Print and shaded views of the part. All mm, measured from the part's lowest x, y and z. A direction names the side the tool comes from. Coordinates: 2 decimals unless noted, no trailing zeros. Loops run counter-clockwise (first coordinate to the right, second up) from the corner with the lowest first, then second, coordinate; pieces in that order, holes last. Notation, with made-up numbers: (-16, -31) -> (1, -31) arc R17 cw to (1, -13) -> close; hole circle Ø4 at (-35, 44.5). An arc over 180 degrees is marked (long way). One line per question, with ' | ' between items. Start each with the question number.
1) Two-plate mould, pull along Z, no slides. Class the marked faces 1, 2 and 3: released by +Z, released by -Z, zero draft, split by the parting line, or undercut.
2) Probe L1, parallel to Y at x = 2.5, z = 6.25; L2, parallel to Z at x = 2.75, y = 3.4; L3, parallel to Z at x = 4.5, y = 2.85. List the from-to ranges inside material, lowest first. Write a range as from..to.
3) Cut at A-A (x = 3.5). List the corners of the cut face in (y, z), plus the area to 3 significant figures.
4) 3-axis set-ups, long thin cutter, end or side, ignore diameter. For the marked faces 4 and 5: which of +Z, -Z, +X, -X, +Y, -Y reach the whole face in a straight line?
5) Cut at B-B (y = 2.35). List the corners of the cut face in (x, z).
6) Cut at D-D (x = 1). List the corners of the cut face in (y, z).
7) Cut at C-C (z = 3.25). List the corners of the cut face in (x, y), plus the area to 3 significant figures.
8) Drop flat-ended pins along their axis: pin 1 (1 mm diameter, centred on x = 6, y = 3.5, fed in from -Z); pin 2 (0.9 mm diameter, centred on x = 3.5, z = 3, fed in from +Y); pin 3 (3 mm diameter, centred on y = 1.5, z = 0.5, fed in from -X). Give the stop position or say it passes through.
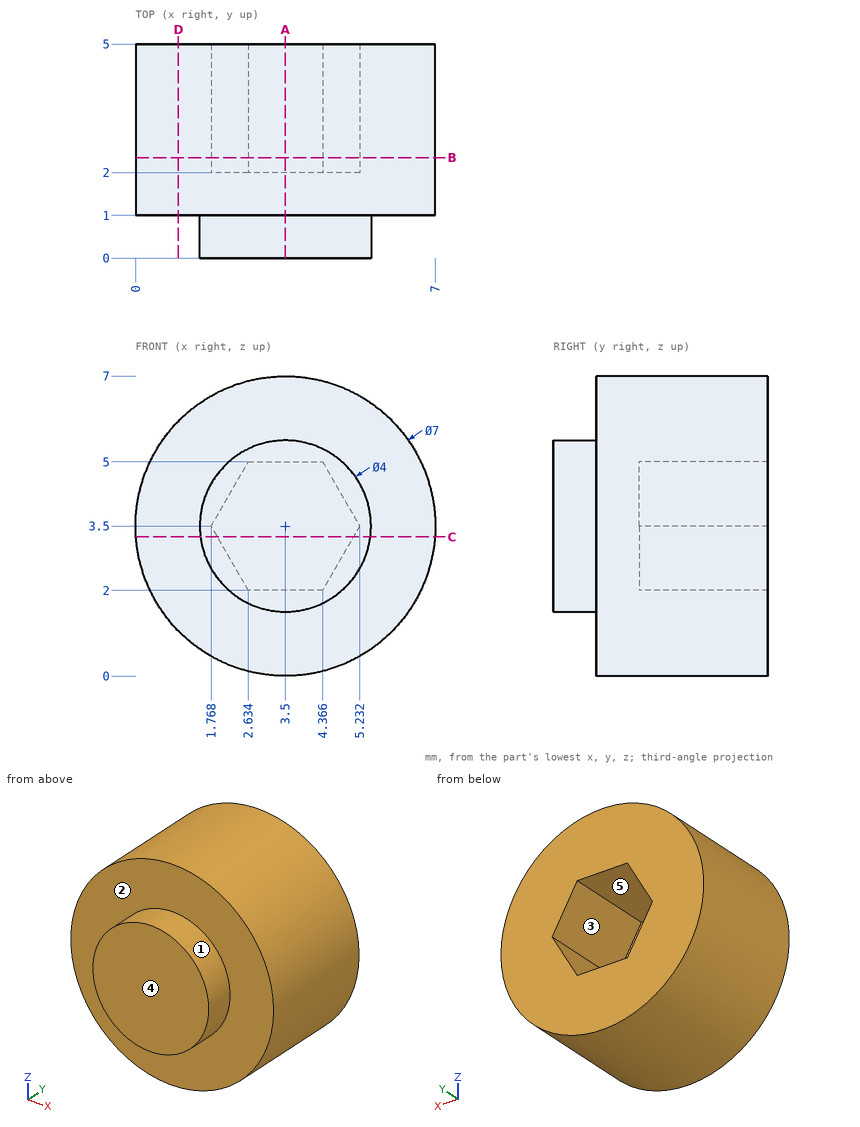
Reported:
1) face 1: split by the parting line | face 2: zero draft | face 3: undercut
2) L1: y = 1..5 | L2: z = 0.08..2, 5..6.92 | L3: z = 0.15..2.23, 4.77..6.85
3) outline: (0, 1.5) -> (1, 1.5) -> (1, 0) -> (5, 0) -> (5, 2) -> (2, 2) -> (2, 5) -> (5, 5) -> (5, 7) -> (1, 7) -> (1, 5.5) -> (0, 5.5) -> close | area: 23.0 mm²
4) face 4: +Z, -Z, +X, -X, -Y | face 5: +Y
5) outline: circle Ø7 at (3.5, 3.5); hole (1.77, 3.5) -> (2.63, 2) -> (4.37, 2) -> (5.23, 3.5) -> (4.37, 5) -> (2.63, 5) -> close
6) outline: (1, 1.05) -> (5, 1.05) -> (5, 5.95) -> (1, 5.95) -> close
7) outline: (0.01, 1) -> (1.52, 1) -> (1.52, 0) -> (5.48, 0) -> (5.48, 1) -> (6.99, 1) -> (6.99, 5) -> (5.09, 5) -> (5.09, 2) -> (1.91, 2) -> (1.91, 5) -> (0.01, 5) -> close | area: 22.4 mm²
8) pin 1: stops at z = 0.63 | pin 2: stops at y = 2 | pin 3: stops at x = 0.34
